```python
from build123d import *

# Parameters (mm, degrees)
ESQUISSE1_R             = 30
BOSS_EXTRU_1_DEPTH      = 27
ESQUISSE3_R             = 21
ENL_V_MAT_EXTRU_1_DEPTH = 10
ENL_V_START             = -10
ESQUISSE4_R             = 21
ENL_V_MAT_EXTRU_2_DEPTH = 10
ESQUISSE5_R             = 10
ENL_V_MAT_EXTRU_3_DEPTH = 10


with BuildPart() as part:
    # Esquisse1 → Boss.-Extru.1 (new body)
    with BuildSketch(Plane.XY):
        Circle(ESQUISSE1_R)
    extrude(amount=BOSS_EXTRU_1_DEPTH)

    # Esquisse3 → Enlèv. mat.-Extru.1 (cut)
    with BuildSketch(Plane.XY.offset(27)):
        Circle(ESQUISSE3_R)
    extrude(amount=-ENL_V_MAT_EXTRU_1_DEPTH, mode=Mode.SUBTRACT)

    # Esquisse4 → Enlèv. mat.-Extru.2 (cut)
    with BuildSketch(Plane(origin=(0, 0, 0), x_dir=(-1, 0, 0), z_dir=(0, 0, -1)).offset(ENL_V_START)):
        with Locations(Location((0, 0, 0), (0, 0, 180))):
            Circle(ESQUISSE4_R)
    extrude(amount=ENL_V_MAT_EXTRU_2_DEPTH, mode=Mode.SUBTRACT)

    # Esquisse5 → Enlèv. mat.-Extru.3 (cut)
    with BuildSketch(Plane(origin=(0, 0, 10), x_dir=(-1, 0, 0), z_dir=(0, 0, -1))):
        Circle(ESQUISSE5_R)
    extrude(amount=-ENL_V_MAT_EXTRU_3_DEPTH, mode=Mode.SUBTRACT)


solid = part.part
```
CAD build for the part. Positions are in the model's coordinates, mm. A direction names the side the tool comes from. Round coordinates to 2 decimals unless told otherwise and drop trailing zeros. Order: outer loops, then holes, each group sorted by start corner. A loop starts at its lowest first (then second) coordinate and runs counter-clockwise, first axis right, second up.
Q1. Which spindle directions (+Z, -Z, +X, -X, +Y, -Y) get a long thin tool onto all of the face, cutting with end or side? Do faces 4 (the flat face through (9, 5, 17)), 5 (the cylindrical face through (20.03, -6.31, 5.07)), 6 (the cylindrical face through (2.17, -9.76, 13.45)). Say none if no direction does.
Q2. Slice it at C-C (y = -17). Write the cut outline in (x, z).
Q3. Two-plate mould, pull along X, no slides. Class faces 1 (the cylindrical face through (-29.97, 1.32, 13.31)), 2 (the cylindrical face through (20.03, 6.31, 22.07)), 3 (the flat face through (6.2, 20.4, 27)): pulls with the +X half, pulls with the -X half, needs draft (parallel to the pull), parting line crosses it, or undercut.
Q4. Drop flat-ended pins along their axis: pin 1 (21 mm diameter, centred on x = 3, y = -2, fed in from -Z); pin 2 (2 mm diameter, centred on x = -6, z = 9, fed in from -Y); pin 3 (5 mm diameter, centred on x = 15.5, z = 21, fed in from -Y). Give the stop position or say it passes through.
Q5. Slice it at D-D (z = 5). Write the cut outline in (x, y), and give its area (3 significant figures).
Q6. Slice it at A-A (x = 0). Write the cut outline in (y, z).
Q7. Wall check: L1, parallel to Y at x = 0, z = 13.5; L2, parallel to X at y = -11, z = 21.75; L3, parallel to Z at x = 7, y = -18. Give the ranges that are in metal, low to high.
Results below:
1. face 4: +Z
1. face 5: -Z
1. face 6: +Z, -Z
2. outline: (-24.72, 0) - (-12.33, 0) - (-12.33, 10) - (12.33, 10) - (12.33, 0) - (24.72, 0) - (24.72, 27) - (12.33, 27) - (12.33, 17) - (-12.33, 17) - (-12.33, 27) - (-24.72, 27) - close
3. face 1: parting line crosses it
3. face 2: undercut
3. face 3: needs draft
4. pin 1: stops at z = 10
4. pin 2: stops at y = -29.58
4. pin 3: stops at y = -27.04
5. outline: circle Ø60 at (0, 0); hole circle Ø42 at (0, 0)
5. area: 1,440 mm2
6. outline: (-30, 0) - (-21, 0) - (-21, 10) - (-10, 10) - (-10, 17) - (-21, 17) - (-21, 27) - (-30, 27) - close; (10, 10) - (21, 10) - (21, 0) - (30, 0) - (30, 27) - (21, 27) - (21, 17) - (10, 17) - close
7. L1: y = -30 to -10, 10 to 30
7. L2: x = -27.91 to -17.89, 17.89 to 27.91
7. L3: z = 10 to 17
